Can you work these out from the model? Positions are in its coordinate system, mm. Face numbers are marked on the shaded views. A direction names the side the tool comes from. Coordinates: 2 decimals unless noted, no trailing zeros. Order: outer loops, then holes, each group sorted by start corner. A loop starts at its lowest first (then second) coordinate and runs counter-clockwise, first axis right, second up. Notation, with made-up numbers: (-26, 66) -> (28, 66) arc R25 cw to (28, 91) -> close; hole circle Ø6 at (0.5, 37.25). An arc over 180 degrees is marked (long way). Return JSON: item names as keys, results as strings. Group by question number.
1) For the marked faces 1, 2 and 3, which set-ups out of +Z, -Z, +X, -X, +Y, -Y let a thin tool reach every point of the face, with its end or its side?
2) If I drill on probe 1 along X at (y, z) = (27, 0); probe 2 along Z at (x, y) = (-5.25, 19); probe 3 along Y at (x, z) = (4.25, 11), over which ranges is the centre line in solid material (lowest first)? Write a range as from..to.
3) If we section it at A-A, the plane z = 0: Please give me the cut outline in (x, y) (3 decimals), then the cut area to 3 significant figures.
4) If we section it at C-C, the plane y = 29: Please give me the cut outline in (x, z).
5) If we section it at B-B, the plane y = 45.5: Please give me the cut outline in (x, z) (3 decimals).
6) For pin 1 (1.5 mm diameter, centred on x = 6, z = 10.5, fed in from +Y); pin 2 (5 mm diameter, centred on y = 22.5, z = 8, fed in from -X); pin 3 (6 mm diameter, centred on x = 11, y = 20, fed in from +Z); pin 4 (8 mm diameter, centred on x = 2, z = -3.5, fed in from +Y), each with a flat end and sliding along its axis, tell me the tip position at first contact or that it passes through.
7) Thinking about a two-plate mould opening in X: for the marked faces 4, 5 and 6, which applies, +X half, -X half, draft (parallel to the pull), parting line (faces both ways), or undercut?
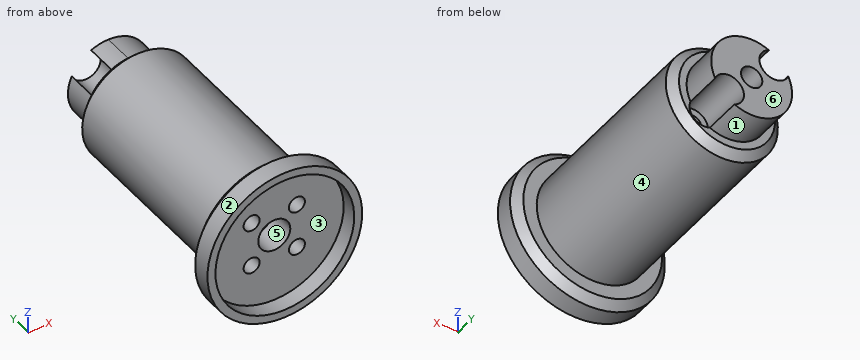
from build123d import *

# Parameters (mm, degrees)
SKETCH1_R              = 14.5
BOSS_EXTRUDE1_DEPTH    = 5
SKETCH2_R              = 13
CUT_EXTRUDE1_DEPTH     = 3
SKETCH6_R              = 10.5
BOSS_EXTRUDE3_DEPTH    = 45.2
CUT_EXTRUDE2_START     = -2
SKETCH3_R              = 3
SKETCH3_R_2            = 1.5
CUT_EXTRUDE2_DEPTH     = 5
BEARING_START          = -7
SKETCH7_R              = 10.5
SKETCH7_R_2            = 7.575
BEARING_SUPPORT_DEPTH  = 7
SKETCH8_R              = 2
SKETCH8_R_2            = 1.5
M4_HOLE_BORE_DEPTH     = 52.462024834
SKETCH9_R              = 2.8
M3_BOLT_RECESSES_DEPTH = 10.2
CHAMFER1_SIZE          = 1.5


with BuildPart() as part:
    # Sketch1 → Boss-Extrude1 (new body)
    with BuildSketch(Plane(origin=(0, 0, 0), x_dir=(1, 0, 0), z_dir=(0, 1, 0))):
        with Locations(Location((0, 0, 0), (0, 0, 270))):
            Circle(SKETCH1_R)
    extrude(amount=BOSS_EXTRUDE1_DEPTH)

    # Sketch2 → Cut-Extrude1 (cut)
    with BuildSketch(Plane.XZ):
        with Locations(Location((0, 0, 0), (0, 0, 270))):
            Circle(SKETCH2_R)
    extrude(amount=-CUT_EXTRUDE1_DEPTH, mode=Mode.SUBTRACT)

    # Sketch6 → Boss-Extrude3 (add)
    with BuildSketch(Plane(origin=(0, 5, 0), x_dir=(1, 0, 0), z_dir=(0, 1, 0))):
        with Locations(Location((0, 0, 0), (0, 0, 270))):
            Circle(SKETCH6_R)
    extrude(amount=BOSS_EXTRUDE3_DEPTH)

    # Sketch3 → Cut-Extrude2 (cut)
    with BuildSketch(Plane(origin=(0, 5, 0), x_dir=(1, 0, 0), z_dir=(0, 1, 0)).offset(CUT_EXTRUDE2_START)):
        with Locations(Location((0, 0, 0), (0, 0, 90))):
            Circle(SKETCH3_R)
        with Locations(Location((-4.242640687, 4.242640687, 0), (0, 0, 90))):
            Circle(SKETCH3_R_2)
        with Locations(Location((4.242640687, 4.242640687, 0), (0, 0, 90))):
            Circle(SKETCH3_R_2)
        with Locations(Location((4.242640687, -4.242640687, 0), (0, 0, 90))):
            Circle(SKETCH3_R_2)
        with Locations(Location((-4.242640687, -4.242640687, 0), (0, 0, 90))):
            Circle(SKETCH3_R_2)
    extrude(amount=CUT_EXTRUDE2_DEPTH, mode=Mode.SUBTRACT)

    # Sketch7 → Bearing Support (cut)
    with BuildSketch(Plane(origin=(0, 50.2, 0), x_dir=(1, 0, 0), z_dir=(0, 1, 0)).offset(BEARING_START)):
        with Locations(Location((0, 0, 0), (0, 0, 270))):
            Circle(SKETCH7_R)
        with Locations(Location((0, 0, 0), (0, 0, 270))):
            Circle(SKETCH7_R_2, mode=Mode.SUBTRACT)
    extrude(amount=BEARING_SUPPORT_DEPTH, mode=Mode.SUBTRACT)

    # Sketch8 → M4 Hole Bore (cut, through all)
    with BuildSketch(Plane.XZ.offset(-3)):
        with Locations(Location((0, 0, 0), (0, 0, 270))):
            Circle(SKETCH8_R)
        with Locations(Location((-4.242640687, 4.242640687, 0), (0, 0, 270))):
            Circle(SKETCH8_R_2)
        with Locations(Location((4.242640687, -4.242640687, 0), (0, 0, 270))):
            Circle(SKETCH8_R_2)
    extrude(amount=-M4_HOLE_BORE_DEPTH, mode=Mode.SUBTRACT)

    # Sketch9 → M3 Bolt Recesses (cut)
    with BuildSketch(Plane(origin=(0, 50.2, 0), x_dir=(1, 0, 0), z_dir=(0, 1, 0))):
        with Locations(Location((4.242640687, 4.242640687, 0), (0, 0, 270))):
            Circle(SKETCH9_R)
        with Locations(Location((-4.242640687, -4.242640687, 0), (0, 0, 270))):
            Circle(SKETCH9_R)
    extrude(amount=-M3_BOLT_RECESSES_DEPTH, mode=Mode.SUBTRACT)

    # Chamfer1
    chamfer1_edges = [part.edges().sort_by_distance(p)[0] for p in [
        (0, 43.2, -10.5),
        (0, 5, -14.5),
    ]]
    chamfer(chamfer1_edges, length=CHAMFER1_SIZE)


solid = part.part
Result sheet:
{
 "1": {"face 1": "+Y", "face 2": "+Y, -Y", "face 3": "-Y"},
 "2": {"probe 1": "x = -10.5..-2, 2..10.5", "probe 2": "z = -9.09..3.13, 5.35..9.09", "probe 3": "y = 3..5"},
 "3": {"outline": "(-14.5, 0) -> (-13, 0) -> (-13, 3) -> (-3, 3) -> (-3, 8) -> (-2, 8) -> (-2, 50.2) -> (-7.575, 50.2) -> (-7.575, 43.2) -> (-9, 43.2) -> (-10.5, 41.7) -> (-10.5, 5) -> (-13, 5) -> (-14.5, 3.5) -> close; (2, 8) -> (3, 8) -> (3, 3) -> (13, 3) -> (13, 0) -> (14.5, 0) -> (14.5, 3.5) -> (13, 5) -> (10.5, 5) -> (10.5, 41.7) -> (9, 43.2) -> (7.575, 43.2) -> (7.575, 50.2) -> (2, 50.2) -> close", "area": "772 mm2"},
 "4": {"outline": "circle Ø21 at (0, 0); hole circle Ø3 at (-4.24, 4.24); hole circle Ø4 at (0, 0); hole circle Ø3 at (4.24, -4.24)"},
 "5": {"outline": "(-6.853, 3.229) arc R7.575 ccw to (3.229, -6.853) arc R2.8 cw (long way) to (6.853, -3.229) arc R7.575 ccw to (-3.229, 6.853) arc R2.8 cw (long way) to start; hole circle Ø4 at (0, 0)"},
 "6": {"pin 1": "stops at y = 5", "pin 2": "stops at x = -8.94", "pin 3": "stops at z = 6.8", "pin 4": "stops at y = 50.2"},
 "7": {"face 4": "parting line", "face 5": "undercut", "face 6": "draft"}
}
